Verification items for the finished model (mm, model axes). A direction names the side the tool comes from. Round coordinates to 2 decimals unless told otherwise and drop trailing zeros. Write each loop counter-clockwise with the first axis right and the second up, starting at its lowest first coordinate (ties: lowest second). Pieces come first, ordered by that corner, then holes. Notation, with made-up numbers: M -4.5,70.5 L 29.5,70.5 A15 cw 29.5,97.5 Z; hole C 24.5,-3 d2. An arc over 180 degrees is marked long. Answer in a Markdown table with one row per item. Add a question column.
1. Draft check along X on faces 1 (the flat face through (1, 4.315, 3)), 2 (the flat face through (33.217, -8, 3)), 3 (the flat face through (19, -5.21, 3)). Enter one of: pulls with the +X half, pulls with the -X half, needs draft (parallel to the pull), parting line crosses it, or undercut.
2. Sectioned sample at A-A on y = -13.5. Record the cut outline in (x, z).
3. Material ranges on probe 1 along Y at (x, z) = (25, 2); probe 2 along X at (y, z) = (-14.5, 2); probe 3 along Y at (x, z) = (2.5, 4.75), recorded low to high.
4. Set-up check for faces 4 (the flat face through (4.363, -15, 3)), 5 (the flat face through (-30.283, -2, 3)), 6 (the flat face through (19, -16.64, 3)): record each of +Z, -Z, +X, -X, +Y, -Y from which the full face is reachable in a straight line by a thin tool's end or side.
5. Sectioned sample at B-B on x = 14. Record the cut outline in (y, z).
6. Go/stop test with flat-tipped pins: pin 1 Ø3 at (y, z) = (-17.5, 4) entering from -X; pin 2 Ø3 at (x, y) = (-23.93, -2.03) entering from -Z; pin 3 Ø2 at (x, z) = (-23.5, 2) entering from -Y. Record where each tip stops, or that it passes through.
7. Sectioned sample at D-D on z = 5. Record the cut outline in (x, y) (1 decimal).
8. Sectioned sample at C-C on x = -23. Record the cut outline in (y, z), plus the area to 3 significant figures.
```python
from build123d import *

# Parameters (mm, degrees)
BOSS_EXTRUDE1_DEPTH = 6.35
SKETCH2_R           = 1.5875
SKETCH2_W           = 18.214797942
SKETCH2_H           = 5.08
SKETCH2_W_2         = 18.693309481
CUT_EXTRUDE1_DEPTH  = 6.35


with BuildPart() as part:
    # Sketch1 → Boss-Extrude1 (new body)
    with BuildSketch(Plane.XY):
        Polygon((-30.283460543, 4.315489798), (33.216539457, 4.315489798), (33.216539457, -21.084510202), (4.363229976, -21.084510202), (4.363229976, -8.384510202), (-30.283460543, -8.384510202), align=None)
    extrude(amount=BOSS_EXTRUDE1_DEPTH)

    # Sketch2 → Cut-Extrude1 (cut)
    with BuildSketch(Plane.XY.offset(6.35)):
        with Locations((-23.933460543, -2.034510202)):
            Circle(SKETCH2_R)
        with Locations((1.466539457, -2.034510202)):
            Circle(SKETCH2_R)
        with Locations((19.029140486, -2.669510202)):
            Rectangle(SKETCH2_W, SKETCH2_H)
        with Locations((18.789884717, -14.099510202)):
            Rectangle(SKETCH2_W_2, SKETCH2_H)
    extrude(amount=-CUT_EXTRUDE1_DEPTH, mode=Mode.SUBTRACT)


solid = part.part
```
Geometry check:
| question | item | result |
|---|---|---|
| 1 | face 1 | needs draft |
| 1 | face 2 | pulls with the +X half |
| 1 | face 3 | undercut |
| 2 | outline | M 4.36,0 L 9.44,0 L 9.44,6.35 L 4.36,6.35 Z; M 28.14,0 L 33.22,0 L 33.22,6.35 L 28.14,6.35 Z |
| 3 | probe 1 | y = -21.08 to -16.64, -11.56 to -5.21, -0.13 to 4.32 |
| 3 | probe 2 | x = 4.36 to 9.44, 28.14 to 33.22 |
| 3 | probe 3 | y = -8.38 to -3.24, -0.83 to 4.32 |
| 4 | face 4 | +Z, -Z, -X, -Y |
| 4 | face 5 | +Z, -Z, -X, +Y, -Y |
| 4 | face 6 | +Z, -Z |
| 5 | outline | M -21.08,0 L -16.64,0 L -16.64,6.35 L -21.08,6.35 Z; M -11.56,0 L -5.21,0 L -5.21,6.35 L -11.56,6.35 Z; M -0.13,0 L 4.32,0 L 4.32,6.35 L -0.13,6.35 Z |
| 6 | pin 1 | stops at x = 4.36 |
| 6 | pin 2 | passes through |
| 6 | pin 3 | stops at y = -8.38 |
| 7 | outline | M -30.3,-8.4 L 4.4,-8.4 L 4.4,-21.1 L 33.2,-21.1 L 33.2,4.3 L -30.3,4.3 Z; hole C -23.9,-2 d3.2; hole C 1.5,-2 d3.2; hole M 9.4,-16.6 L 28.1,-16.6 L 28.1,-11.6 L 9.4,-11.6 Z; hole M 9.9,-5.2 L 28.1,-5.2 L 28.1,-0.1 L 9.9,-0.1 Z |
| 8 | outline | M -8.38,0 L -3.32,0 L -3.32,6.35 L -8.38,6.35 Z; M -0.75,0 L 4.32,0 L 4.32,6.35 L -0.75,6.35 Z |
| 8 | area | 64.3 mm2 |
